Design review of the part built by this model. Coordinates are the model's own, in mm. Give positions to 0.01 mm unless a question says otherwise; leave off trailing zeros. Order: outer loops, then holes, each group sorted by start corner. A loop starts at its lowest first (then second) coordinate and runs counter-clockwise, first axis right, second up. Notation, with made-up numbers: (60, -10) -> (108, -10) arc R32 ccw to (108, 26) -> close; hole circle Ø2 at (3, 16). An arc over 180 degrees is marked (long way). One line per item, written item: value.
from build123d import *

# Parameters (mm, degrees)
SKETCH1_W                = 136
SKETCH1_H                = 77
SKETCH1_R                = 1.725
BOSS_EXTRUDE1_DEPTH      = 7.85
BOSS_EXTRUDE1_DEPTH_BACK = 6
SKETCH2_W                = 107
SKETCH2_H                = 77
BOSS_EXTRUDE2_DEPTH      = 29
CUT_EXTRUDE1_DEPTH       = 32.5
SKETCH4_W                = 2
SKETCH4_H                = 8
BOSS_EXTRUDE3_DEPTH      = 32.5
FILLET1_R                = 5
FILLET4_R                = 1


with BuildPart() as part:
    # Sketch1 → Boss-Extrude1 (new body, two sides)
    with BuildSketch(Plane.XY) as boss_extrude1_sk:
        Rectangle(SKETCH1_W, SKETCH1_H)
        with Locations((-58.35, 0)):
            Circle(SKETCH1_R, mode=Mode.SUBTRACT)
        with Locations((58.35, 0)):
            Circle(SKETCH1_R, mode=Mode.SUBTRACT)
    extrude(amount=BOSS_EXTRUDE1_DEPTH)
    extrude(boss_extrude1_sk.sketch, amount=-BOSS_EXTRUDE1_DEPTH_BACK)

    # Sketch2 → Boss-Extrude2 (add)
    with BuildSketch(Plane(origin=(0, 0, -6), x_dir=(-1, 0, 0), z_dir=(0, 0, -1))):
        Rectangle(SKETCH2_W, SKETCH2_H)
    extrude(amount=BOSS_EXTRUDE2_DEPTH)

    # Sketch3 → Cut-Extrude1 (cut)
    with BuildSketch(Plane.XY.offset(7.85)):
        Polygon((-38.95, 33.85), (-38.95, 25.85), (-40.95, 25.85), (-40.95, 33.85), (-50.35, 33.85), (-50.35, 1.75), (50.25, 1.75), (50.25, 33.85), (40.85, 33.85), (40.85, 25.85), (38.85, 25.85), (38.85, 33.85), (29.45, 33.85), (29.45, 25.85), (27.45, 25.85), (27.45, 33.85), (18.05, 33.85), (18.05, 25.85), (16.05, 25.85), (16.05, 33.85), (6.65, 33.85), (6.65, 25.85), (4.65, 25.85), (4.65, 33.85), (-4.75, 33.85), (-4.75, 25.85), (-6.75, 25.85), (-6.75, 33.85), (-16.15, 33.85), (-16.15, 25.85), (-18.15, 25.85), (-18.15, 33.85), (-27.55, 33.85), (-27.55, 25.85), (-29.55, 25.85), (-29.55, 33.85), align=None)
    cut_extrude1 = extrude(amount=-CUT_EXTRUDE1_DEPTH, mode=Mode.SUBTRACT)

    # Mirror1: Cut-Extrude1 across plane
    add(cut_extrude1.mirror(Plane.ZX), mode=Mode.SUBTRACT)

    # Sketch4 → Boss-Extrude3 (add)
    with BuildSketch(Plane.XY.offset(7.85)):
        with Locations((-39.95, 5.75)):
            Rectangle(SKETCH4_W, SKETCH4_H)
        with Locations((-28.55, 5.75)):
            Rectangle(SKETCH4_W, SKETCH4_H)
        with Locations((-17.15, 5.75)):
            Rectangle(SKETCH4_W, SKETCH4_H)
        with Locations((-5.75, 5.75)):
            Rectangle(SKETCH4_W, SKETCH4_H)
        with Locations((5.65, 5.75)):
            Rectangle(SKETCH4_W, SKETCH4_H)
        with Locations((17.05, 5.75)):
            Rectangle(SKETCH4_W, SKETCH4_H)
        with Locations((28.45, 5.75)):
            Rectangle(SKETCH4_W, SKETCH4_H)
        with Locations((39.85, 5.75)):
            Rectangle(SKETCH4_W, SKETCH4_H)
    boss_extrude3 = extrude(amount=-BOSS_EXTRUDE3_DEPTH)

    # Mirror2: Boss-Extrude3 across plane
    add(boss_extrude3.mirror(Plane.ZX))

    # Fillet1
    fillet1_edges = [part.edges().sort_by_distance(p)[0] for p in [
        (-68, 38.5, 0.925),
        (68, 38.5, 0.925),
        (68, -38.5, 0.925),
        (-68, -38.5, 0.925),
    ]]
    fillet(fillet1_edges, radius=FILLET1_R)

    # Fillet4
    fillet4_edges = [part.edges().sort_by_distance(p)[0] for p in [
        (53.5, 38.5, -20.5),
        (53.5, -38.5, -20.5),
        (-53.5, -38.5, -20.5),
        (-53.5, 38.5, -20.5),
        (53.5, 0, -35),
        (0, -38.5, -35),
        (-53.5, 0, -35),
        (0, 38.5, -35),
    ]]
    fillet(fillet4_edges, radius=FILLET4_R)


solid = part.part
Item 1: Add section A-A on x = 58.35. Give the boundary of the cut face in (y, z) (3 decimals).
Returned:
outline: (-38.5, -6) -> (-1.725, -6) -> (-1.725, 7.85) -> (-38.5, 7.85) -> close; (1.725, -6) -> (38.5, -6) -> (38.5, 7.85) -> (1.725, 7.85) -> close
Item 2: Clearance check with flat-ended pins moving along their axes: P1, Ø4, axis at y = -13.5, z = -10, coming from the -X side; P2, Ø3, axis at x = 26.5, y = 11.5, coming from the +Z side; P3, Ø8, axis at y = 30, z = -29.5, coming from the +X side. State where each tip first meets the part, or that it passes through.
Returned:
P1: x = -53.5
P2: z = -24.65
P3: x = 53.5
Item 3: To check wall thickness, follow line 1 along Y through (x, z) = (5.5, -3); line 2 along Y through (x, z) = (-1, -15.5); line 3 along Y through (x, z) = (-58.35, 5.5) (3 decimals). State the ranges of each line that lie inside material, in increasing order. Write a range as from..to.
Returned:
line 1: -38.5..-25.85, -9.75..9.75, 25.85..38.5
line 2: -38.5..-33.85, -1.75..1.75, 33.85..38.5
line 3: -38.5..-1.725, 1.725..38.5
Item 4: Draft analysis for pull direction X (two halves, no side actions). For faces 1 (the cylindrical face through (66.5, 37.07, 0.83)), 2 (the flat face through (6.65, 6, -8)), 3 (the flat face through (23, -1.75, -8)), state which applies: pulls with the +X half, pulls with the -X half, needs draft (parallel to the pull), parting line crosses it, or undercut.
Returned:
face 1: pulls with the +X half
face 2: undercut
face 3: undercut
Item 5: Add section D-D on y = 18.5. Give the boundary of the cut face in (x, z).
Returned:
outline: (-68, -6) -> (-53.5, -6) -> (-53.5, -34) arc R1 ccw to (-52.5, -35) -> (52.5, -35) arc R1 ccw to (53.5, -34) -> (53.5, -6) -> (68, -6) -> (68, 7.85) -> (50.25, 7.85) -> (50.25, -24.65) -> (-50.35, -24.65) -> (-50.35, 7.85) -> (-68, 7.85) -> close
Item 6: Add section B-B on y = 0. Give the boundary of the cut face in (x, z) (3 decimals), plus the area to 3 significant figures.
Returned:
outline: (-68, -6) -> (-60.075, -6) -> (-60.075, 7.85) -> (-68, 7.85) -> close; (-56.625, -6) -> (-53.5, -6) -> (-53.5, -34) arc R1 ccw to (-52.5, -35) -> (52.5, -35) arc R1 ccw to (53.5, -34) -> (53.5, -6) -> (56.625, -6) -> (56.625, 7.85) -> (-56.625, 7.85) -> close; (60.075, -6) -> (68, -6) -> (68, 7.85) -> (60.075, 7.85) -> close
area: 4,890 mm²
Item 7: Add section C-C on x = 1.5. Give the boundary of the cut face in (y, z).
Returned:
outline: (-38.5, -34) arc R1 ccw to (-37.5, -35) -> (37.5, -35) arc R1 ccw to (38.5, -34) -> (38.5, 7.85) -> (33.85, 7.85) -> (33.85, -24.65) -> (1.75, -24.65) -> (1.75, 7.85) -> (-1.75, 7.85) -> (-1.75, -24.65) -> (-33.85, -24.65) -> (-33.85, 7.85) -> (-38.5, 7.85) -> close
